Read the model definition and answer for the solid it produces. Units are mm, in the model's axes. Face numbers are marked on the shaded views. A direction names the side the tool comes from. Round coordinates to 2 decimals unless told otherwise and drop trailing zeros. Order: outer loops, then holes, each group sorted by start corner. A loop starts at its lowest first (then second) coordinate and runs counter-clockwise, first axis right, second up. Notation, with made-up numbers: (-35.5, -2) - (9.5, -2) arc R20 ccw to (9.5, 7) - close; hole circle Ø7 at (48, -34.75). An arc over 180 degrees is marked (long way). One line per question, with ' | ' between items. Start each with the question number.
1) The part is cut by section C-C, the plane y = 11. Give the vertices of the cut face in (x, z), plus the area to 3 significant figures.
2) The part is cut by section B-B, the plane z = 0. Give the vertices of the cut face in (x, y), plus the area to 3 significant figures.
3) The mould has two halves that part along Y. Classify the marked faces 1, 2 and 3: pulls with the +Y half, pulls with the -Y half, needs draft (parallel to the pull), parting line crosses it, or undercut.
4) For the marked faces 4, 5, 6, 7 and 8, determine the directions among +Z, -Z, +X, -X, +Y, -Y from which every point of the face is accessible in a straight line to the end or side of a thin tool.
5) The part is cut by section A-A, the plane x = 4.5. Give the vertices of the cut face in (y, z).
6) A flat-ended cylindrical pin translates along its axis: pin 1 (1.4 mm diameter, centred on y = 9, z = -0.5, fed in from +X). Find the tip coordinate at first contact, or state that the pin passes through.
7) Straight lines are drawn through the part: line 1 (X direction, y = 7.75, z = -1.25); line 2 (Y direction, x = 2, z = 6.5); line 3 (X direction, y = 0.5, z = 0). For each, find the intervals that lie inside material, in ascending order. Write a range as from..to.
8) The part is cut by section D-D, the plane x = 0. Give the vertices of the cut face in (y, z), plus the area to 3 significant figures.
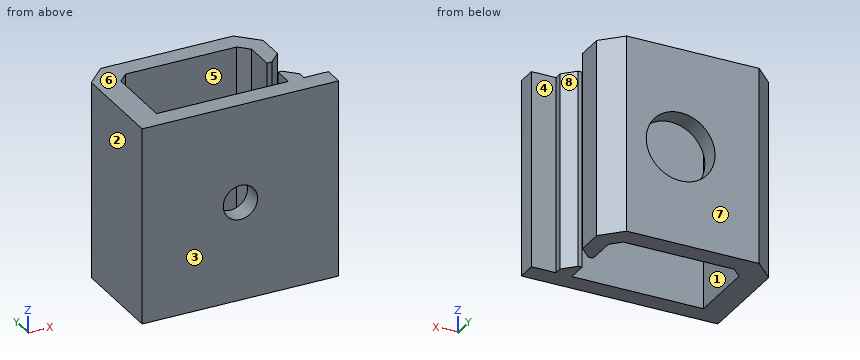
from build123d import *

# Parameters (mm, degrees)
SKETCH1_W           = 20
SKETCH1_H           = 20
SKETCH1_R           = 1.75
BOSS_EXTRUDE1_DEPTH = 2
SKETCH2_W           = 2.5
SKETCH2_H           = 20
BOSS_EXTRUDE2_DEPTH = 10
SKETCH3_W           = 20
SKETCH3_H           = 2
BOSS_EXTRUDE3_DEPTH = 15
SKETCH4_W           = 1.7
SKETCH4_H           = 20
BOSS_EXTRUDE4_DEPTH = 4
CHAMFER1_SIZE       = 1.2
CHAMFER2_SIZE       = 2
CHAMFER3_SIZE       = 1
SKETCH5_R           = 1.75
CUT_EXTRUDE1_DEPTH  = 34
SKETCH6_R           = 3.5
CUT_EXTRUDE2_DEPTH  = 2
SKETCH7_W           = 1.6
SKETCH7_H           = 20
BOSS_EXTRUDE5_DEPTH = 2
CHAMFER4_SIZE       = 1.2


with BuildPart() as part:
    # Sketch1 → Boss-Extrude1 (new body)
    with BuildSketch(Plane(origin=(0, 0, 0), x_dir=(1, 0, 0), z_dir=(0, 1, 0))):
        Rectangle(SKETCH1_W, SKETCH1_H)
        with Locations(Location((0, 0, 0), (0, 0, 270))):
            Circle(SKETCH1_R, mode=Mode.SUBTRACT)
    extrude(amount=BOSS_EXTRUDE1_DEPTH)

    # Sketch2 → Boss-Extrude2 (add)
    with BuildSketch(Plane(origin=(0, 2, 0), x_dir=(1, 0, 0), z_dir=(0, 1, 0))):
        with Locations((-8.75, 0)):
            Rectangle(SKETCH2_W, SKETCH2_H)
    extrude(amount=BOSS_EXTRUDE2_DEPTH)

    # Sketch3 → Boss-Extrude3 (add)
    with BuildSketch(Plane(origin=(-7.5, 0, 0), x_dir=(0, 0, -1), z_dir=(1, 0, 0))):
        with Locations((0, 11)):
            Rectangle(SKETCH3_W, SKETCH3_H)
    extrude(amount=BOSS_EXTRUDE3_DEPTH)

    # Sketch4 → Boss-Extrude4 (add)
    with BuildSketch(Plane.XZ.offset(-10)):
        with Locations((6.65, 0)):
            Rectangle(SKETCH4_W, SKETCH4_H)
    extrude(amount=BOSS_EXTRUDE4_DEPTH)

    # Chamfer1
    chamfer1_edges = [part.edges().sort_by_distance(p)[0] for p in [
        (7.5, 6, 0),
    ]]
    chamfer(chamfer1_edges, length=CHAMFER1_SIZE)

    # Chamfer2
    chamfer2_edges = [part.edges().sort_by_distance(p)[0] for p in [
        (-10, 12, 0),
        (7.5, 12, 0),
    ]]
    chamfer(chamfer2_edges, length=CHAMFER2_SIZE)

    # Chamfer3
    chamfer3_edges = [part.edges().sort_by_distance(p)[0] for p in [
        (-7.5, 10, 0),
        (5.8, 10, 0),
    ]]
    chamfer(chamfer3_edges, length=CHAMFER3_SIZE)

    # Sketch5 → Cut-Extrude1 (cut)
    with BuildSketch(Plane.XZ):
        with Locations(Location((0, 0, 0), (0, 0, 90))):
            Circle(SKETCH5_R)
    extrude(amount=-CUT_EXTRUDE1_DEPTH, mode=Mode.SUBTRACT)

    # Sketch6 → Cut-Extrude2 (cut)
    with BuildSketch(Plane(origin=(0, 12, 0), x_dir=(1, 0, 0), z_dir=(0, 1, 0))):
        with Locations(Location((0, 0, 0), (0, 0, 270))):
            Circle(SKETCH6_R)
    extrude(amount=-CUT_EXTRUDE2_DEPTH, mode=Mode.SUBTRACT)

    # Sketch7 → Boss-Extrude5 (add)
    with BuildSketch(Plane(origin=(0, 2, 0), x_dir=(1, 0, 0), z_dir=(0, 1, 0))):
        with Locations((6.7, 0)):
            Rectangle(SKETCH7_W, SKETCH7_H)
    extrude(amount=BOSS_EXTRUDE5_DEPTH)

    # Chamfer4
    chamfer4_edges = [part.edges().sort_by_distance(p)[0] for p in [
        (7.5, 4, 0),
    ]]
    chamfer(chamfer4_edges, length=CHAMFER4_SIZE)


solid = part.part
Values:
1) outline: (-9, -10) - (6.5, -10) - (6.5, 10) - (-9, 10) - close; hole circle Ø7 at (0, 0) | area: 272 mm^2
2) outline: (-10, 0) - (-1.75, 0) - (-1.75, 2) - (-7.5, 2) - (-7.5, 9) - (-6.5, 10) - (-3.5, 10) - (-3.5, 12) - (-8, 12) - (-10, 10) - close; (1.75, 0) - (10, 0) - (10, 2) - (7.5, 2) - (7.5, 2.8) - (6.3, 4) - (5.9, 4) - (5.9, 2) - (1.75, 2) - close; (3.5, 10) - (4.8, 10) - (5.8, 9) - (5.8, 6) - (6.3, 6) - (7.5, 7.2) - (7.5, 10) - (5.5, 12) - (3.5, 12) - close | area: 79.6 mm^2
3) face 1: undercut | face 2: needs draft | face 3: pulls with the -Y half
4) face 4: +Z, -Z, +X, +Y | face 5: +Z, -Z | face 6: +Z, +X, -X, +Y, -Y | face 7: +Z, -Z, +X, -X, +Y | face 8: +Z, -Z, +X
5) outline: (0, -10) - (2, -10) - (2, 10) - (0, 10) - close; (10, -10) - (12, -10) - (12, 10) - (10, 10) - close
6) pin 1: stops at x = 7.5
7) line 1: x = -10..-7.5, 5.8..7.5 | line 2: y = 0..2, 10..12 | line 3: x = -10..-1.75, 1.75..10
8) outline: (0, -10) - (2, -10) - (2, -1.75) - (0, -1.75) - close; (0, 1.75) - (2, 1.75) - (2, 10) - (0, 10) - close; (10, -10) - (12, -10) - (12, -3.5) - (10, -3.5) - close; (10, 3.5) - (12, 3.5) - (12, 10) - (10, 10) - close | area: 59.0 mm^2
